from build123d import *

# Parameters (mm, degrees)
SKETCH1_R           = 2
BOSS_EXTRUDE1_DEPTH = 8
CUT_EXTRUDE1_START  = -10
CUT_EXTRUDE1_DEPTH  = 10


# Read off the part's stored shape, not the designer's step: Cut-Extrude1
with BuildPart() as part:
    # Sketch1 → Boss-Extrude1 (new body)
    with BuildSketch(Plane(origin=(0, 0, 0), x_dir=(1, 0, 0), z_dir=(0, 1, 0))):
        with BuildLine():
            Line((-17.960512242, 22.960512242), (17.960512242, 22.960512242))
            ThreePointArc((17.960512242, 22.960512242), (22.960512242, 17.960512242), (17.960512242, 12.960512242))
            Line((17.960512242, 12.960512242), (-17.960512242, 12.960512242))
            ThreePointArc((-17.960512242, 12.960512242), (-22.960512242, 17.960512242), (-17.960512242, 22.960512242))
        make_face()
        with Locations(Location((-17.960512242, 17.960512242, 0), (0, 0, 270))):
            Circle(SKETCH1_R, mode=Mode.SUBTRACT)
        with Locations(Location((17.960512242, 17.960512242, 0), (0, 0, 270))):
            Circle(SKETCH1_R, mode=Mode.SUBTRACT)
    extrude(amount=BOSS_EXTRUDE1_DEPTH)

    # Cut-Extrude1 outline → Cut-Extrude1 (cut)
    with BuildSketch(Plane.XY.offset(-12.960512242).offset(CUT_EXTRUDE1_START)):
        with BuildLine():
            ThreePointArc((3.3, 3.3), (0, 6.6), (-3.3, 3.3))
            Line((-3.3, 3.3), (-3.3, 0))
            Line((-3.3, 0), (3.3, 0))
            Line((3.3, 0), (3.3, 3.3))
        make_face()
    extrude(amount=CUT_EXTRUDE1_DEPTH, mode=Mode.SUBTRACT)


solid = part.part
The model under review builds one solid part; all positions refer to its coordinate system, in mm. A direction names the side the tool comes from. Give positions to 0.01 mm unless a question says otherwise; leave off trailing zeros. Loops run counter-clockwise (first coordinate to the right, second up) from the corner with the lowest first, then second, coordinate; pieces in that order, holes last. Notation, with made-up numbers: (54.5, 61) -> (73.5, 61) arc R19 cw to (73.5, 94) -> close; hole circle Ø11 at (43, 30.25). An arc over 180 degrees is marked (long way). Put each result on its own line as item: value. Start each with the question number.
1. We need section C-C on x = 0. State the section outline as (y, z) points.
2. Clearance check with flat-ended pins moving along their axes: P1, Ø1, axis at y = 3, z = -14, coming from the -X side; P2, Ø3, axis at x = -17.96, z = -17.96, coming from the +Y side; P3, Ø3, axis at y = 3, z = -20.5, coming from the -X side. State where each tip first meets the part, or that it passes through.
3. Mouldability with a two-part tool opening along X and no side actions: class faces 1 (the face through (22.96, 3.94, -18.07)), 2 (the face through (0, 7, -12.961)), 3 (the face through (3.3, 2, -18)) as released by +X, released by -X, zero draft, split by the parting line, or undercut.
4. We need section A-A on y = 7.5. State the section outline as (x, z) points.
5. For faces 4 (the face through (-3.3, 2, -18)), 5 (the face through (16.744, 3.944, -19.548)), list the 3-axis set-ups (+Z, -Z, +X, -X, +Y, -Y) from which the entire face can be reached by the end or side of a thin tool; tool diameter is ignored.
6. Wall thickness on probe 1 along X at (y, z) = (4.75, -19.25); probe 2 along X at (y, z) = (2.25, -13.75); probe 3 along Z at (x, y) = (19.5, 5): over which ranges is each line inside the solid? List them lowest first.
7. We need section B-B on z = -17. State the section outline as (x, y) points.
Determined:
1. outline: (6.6, -22.96) -> (8, -22.96) -> (8, -12.96) -> (6.6, -12.96) -> close
2. P1: x = -21.57
2. P2: through
2. P3: x = -22.85
3. face 1: released by +X
3. face 2: zero draft
3. face 3: undercut
4. outline: (-17.96, -22.96) -> (17.96, -22.96) arc R5 ccw to (17.96, -12.96) -> (-17.96, -12.96) arc R5 ccw to start; hole circle Ø4 at (-17.96, -17.96); hole circle Ø4 at (17.96, -17.96)
5. face 4: +Z, -Z, -Y
5. face 5: +Y, -Y
6. probe 1: -22.79 to -19.49, -16.43 to -2.96, 2.96 to 16.43, 19.49 to 22.79
6. probe 2: -20.66 to -3.3, 3.3 to 20.66
6. probe 3: -22.72 to -19.24, -16.68 to -13.2
7. outline: (-22.87, 0) -> (-19.71, 0) -> (-19.71, 8) -> (-22.87, 8) -> close; (-16.21, 0) -> (-3.3, 0) -> (-3.3, 3.3) arc R3.3 cw to (3.3, 3.3) -> (3.3, 0) -> (16.21, 0) -> (16.21, 8) -> (-16.21, 8) -> close; (19.71, 0) -> (22.87, 0) -> (22.87, 8) -> (19.71, 8) -> close
